Source: CAD feature listing. Evaluate the final solid. Frame: model axes, mm. A direction names the side the tool comes from. Give positions to 0.01 mm unless a question says otherwise; leave off trailing zeros. Loops run counter-clockwise (first coordinate to the right, second up) from the corner with the lowest first, then second, coordinate; pieces in that order, holes last. Notation, with made-up numbers: M -26,-27 L -14,-27 A13 ccw -14,-10 Z; hole C 89.5,-31 d7. An arc over 180 degrees is marked long. Write item = value, one per line.
Autodesk Fusion 360 part; units mm, degrees
sketch "Sketch1" plane through (0, 0, 0) normal (0, 0, 1) x (1, 0, 0)
  line L0 (0, 0) -> (70, 0)
  line L1 (70, 0) -> (70, 150)
  line L2 (70, 150) -> (0, 150)
  line L3 (0, 150) -> (0, 0)
  circle A0 centre (22.5, 25) radius 3.3
  circle A1 centre (47.5, 25) radius 3.3
  circle A2 centre (22.5, 125) radius 3.3
  circle A3 centre (47.5, 125) radius 3.3
  line L4 (22.5, 25) -> (0, 25)
  line L5 (0, 25) -> (31, 25)
  line L6 (31, 25) -> (31, 37.5)
  line L7 (31, 37.5) -> (0, 37.5)
  line L8 (0, 37.5) -> (0, 25)
  line L9 (0, 25) -> (31, 25)
  line L10 (31, 25) -> (31, 12.5)
  line L11 (31, 12.5) -> (0, 12.5)
  line L12 (0, 12.5) -> (0, 25)
  line L13 (70, 37.5) -> (39, 37.5)
  line L14 (39, 37.5) -> (39, 12.5)
  line L15 (39, 12.5) -> (70, 12.5)
  line L16 (70, 12.5) -> (70, 37.5)
  line L17 (70, 137.5) -> (39, 137.5)
  line L18 (39, 137.5) -> (39, 112.5)
  line L19 (39, 112.5) -> (70, 112.5)
  line L20 (70, 112.5) -> (70, 137.5)
  line L21 (0, 137.5) -> (31, 137.5)
  line L22 (31, 137.5) -> (31, 112.5)
  line L23 (31, 112.5) -> (0, 112.5)
  line L24 (0, 112.5) -> (0, 137.5)
  point P0 (22.5, 25)
  point P1 (47.5, 25)
  point P2 (47.5, 125)
  point P3 (22.5, 125)
  dimension "d1" = 70
  dimension "d2" = 150
  dimension "d3" = 25
  dimension "d4" = 22.5
  dimension "d5" = 25
  dimension "d6" = 22.5
  dimension "d7" = 25
  dimension "d8" = 47.5
  dimension "d9" = 25
  dimension "d10" = 22.5
  dimension "d11" = 22.5
  dimension "d12" = 25
  dimension "d13" = 25
  dimension "d14" = 6.6
  dimension "d15" = 6.6
  dimension "d16" = 6.6
  dimension "d17" = 6.6
  dimension "d18" = 31
  dimension "d19" = 12.5
  dimension "d20" = 12.5
  dimension "d21" = 31
  dimension "d22" = 25
  dimension "d23" = 12.5
  dimension "d24" = 31
  dimension "d25" = 25
  dimension "d26" = 31
  dimension "d27" = 25
  dimension "d28" = 12.5
  dimension "d29" = 12.5
extrude "Extrude1" add sketch "Sketch1" along normal blind 50 contours L0 L1 L2 L3 L6 L7 L10 L11 L13 L14 L15 L17 L18 L19 L21 L22 L23
extrude "Extrude2" add sketch "Sketch1" along normal blind 10 contours L3 A0 L4 L5 L9 L10 L11 L12 | L1 L13 L14 L15 L16 | L3 A0 L4 L5 L6 L7 L8 L9 | L1 L17 L18 L19 L20 | L3 L21 L22 L23 L24
extrude "Extrude3" add 4 faces at (63.6, 25, 10) (6.4, 25, 10) (6.4, 125, 10) (63.6, 125, 10) along direction (0, 0, -1) blind 10 start surface through (0, 0, 50) normal (0, 0, 1)
equation "d14 = 6 mm + 0.6 mm"
1. Cut plane D-D, the plane z = 31.5. Return the cut outline in (x, y).
Derived:
outline = M 0,0 L 70,0 L 70,12.5 L 39,12.5 L 39,37.5 L 70,37.5 L 70,112.5 L 39,112.5 L 39,137.5 L 70,137.5 L 70,150 L 0,150 L 0,137.5 L 31,137.5 L 31,112.5 L 0,112.5 L 0,37.5 L 31,37.5 L 31,12.5 L 0,12.5 Z
2. Material intervals for probe 1 along Y at (x, z) = (47.5, 5); probe 2 along Y at (x, z) = (49.5, 11.5); probe 3 along Z at (x, y) = (13.5, 119), sorted ascending. Write a range as from..to.
Derived:
probe_1 = 0..21.7, 28.3..121.7, 128.3..150
probe_2 = 0..12.5, 37.5..112.5, 137.5..150
probe_3 = 0..10, 40..50
3. Cut plane C-C, the plane x = 14. Return the cut outline in (y, z), then the cut area to 3 significant figures.
Derived:
outline = M 0,0 L 150,0 L 150,50 L 0,50 Z; hole M 12.5,10 L 37.5,10 L 37.5,40 L 12.5,40 Z; hole M 112.5,10 L 137.5,10 L 137.5,40 L 112.5,40 Z
area = 6,000 mm²
4. Reachability of faces 1 (the flat face through (35, 76, 50)), 2 (the flat face through (54, 25, 40)), 3 (the flat face through (31, 125, 25)) from +Z, -Z, +X, -X, +Y, -Y: full face, straight path, thin tool, end or side. Return the list, or none.
Derived:
face_1 = +Z, +X, -X, +Y, -Y
face_2 = +X
face_3 = -X
5. Cut plane A-A, the plane x = 22.5. Return the cut outline in (y, z).
Derived:
outline = M 0,0 L 21.7,0 L 21.7,10 L 12.5,10 L 12.5,40 L 21.7,40 L 21.7,50 L 0,50 Z; M 28.3,0 L 121.7,0 L 121.7,10 L 112.5,10 L 112.5,40 L 121.7,40 L 121.7,50 L 28.3,50 L 28.3,40 L 37.5,40 L 37.5,10 L 28.3,10 Z; M 128.3,0 L 150,0 L 150,50 L 128.3,50 L 128.3,40 L 137.5,40 L 137.5,10 L 128.3,10 Z
6. Cut plane B-B, the plane y = 25. Return the cut outline in (x, z).
Derived:
outline = M 0,0 L 19.2,0 L 19.2,10 L 0,10 Z; M 0,40 L 19.2,40 L 19.2,50 L 0,50 Z; M 25.8,0 L 44.2,0 L 44.2,10 L 39,10 L 39,40 L 44.2,40 L 44.2,50 L 25.8,50 L 25.8,40 L 31,40 L 31,10 L 25.8,10 Z; M 50.8,0 L 70,0 L 70,10 L 50.8,10 Z; M 50.8,40 L 70,40 L 70,50 L 50.8,50 Z
7. First-contact query: pin 1 Ø5.5 at (x, y) = (22.5, 125) entering from +Z. Flat tip, straight axial feed; report the tip coordinate or a pass-through.
Derived:
pin_1 = through
8. Pull-direction query (Y, two-part tool) for faces 4 (the flat face through (35, 76, 0)), 5 (the flat face through (35, 150, 25)), 6 (the cylindrical face through (44.881, 27.008, 4.93)); classes: +Y half, -Y half, draft (parallel to the pull), parting line (faces both ways), or undercut.
Derived:
face_4 = draft
face_5 = +Y half
face_6 = undercut
